from build123d import *

# Parameters (mm, degrees)
TUBE_SQUARE_40_X_40_X_3_2_1_DEPTH = 1920
CUT_EXTRUDE1_DEPTH                = 1921.52076271
SKETCH16_R                        = 2
CUT_EXTRUDE2_DEPTH                = 3
SKETCH17_R                        = 2
CUT_EXTRUDE3_DEPTH                = 3


with BuildPart() as part:
    # Sketch15 → Tube (square) 40 X 40 X 3.2(1) (new body)
    with BuildSketch(Plane(origin=(0, 0, 0), x_dir=(-1, 0, 0), z_dir=(0, 1, 0))):
        with BuildLine():
            Line((-13.6, -20), (13.6, -20))
            ThreePointArc((13.6, -20), (18.1254834, -18.1254834), (20, -13.6))
            Line((20, -13.6), (20, 13.6))
            ThreePointArc((20, 13.6), (18.1254834, 18.1254834), (13.6, 20))
            Line((13.6, 20), (-13.6, 20))
            ThreePointArc((-13.6, 20), (-18.1254834, 18.1254834), (-20, 13.6))
            Line((-20, 13.6), (-20, -13.6))
            ThreePointArc((-20, -13.6), (-18.1254834, -18.1254834), (-13.6, -20))
        make_face()
        with BuildLine():
            Line((-13.6, -16.8), (13.6, -16.8))
            ThreePointArc((13.6, -16.8), (15.8627417, -15.8627417), (16.8, -13.6))
            Line((16.8, -13.6), (16.8, 13.6))
            ThreePointArc((16.8, 13.6), (15.8627417, 15.8627417), (13.6, 16.8))
            Line((13.6, 16.8), (-13.6, 16.8))
            ThreePointArc((-13.6, 16.8), (-15.8627417, 15.8627417), (-16.8, 13.6))
            Line((-16.8, 13.6), (-16.8, -13.6))
            ThreePointArc((-16.8, -13.6), (-15.8627417, -15.8627417), (-13.6, -16.8))
        make_face(mode=Mode.SUBTRACT)
    extrude(amount=TUBE_SQUARE_40_X_40_X_3_2_1_DEPTH)

    # Sketch13 → Cut-Extrude1 (cut, through all)
    with BuildSketch(Plane(origin=(0, 0, -20), x_dir=(-1, 0, 0), z_dir=(0, 0, -1))):
        Polygon((20, 1880), (-20, 1920), (20, 1920), align=None)
    extrude(amount=-CUT_EXTRUDE1_DEPTH, mode=Mode.SUBTRACT)

    # Sketch16 → Cut-Extrude2 (cut)
    with BuildSketch(Plane(origin=(20, 0, 0), x_dir=(0, 0, -1), z_dir=(1, 0, 0))):
        with Locations((0, 1900)):
            Circle(SKETCH16_R)
        with Locations((0, 1447)):
            Circle(SKETCH16_R)
        with Locations((0, 1067)):
            Circle(SKETCH16_R)
        with Locations((0, 687)):
            Circle(SKETCH16_R)
    extrude(amount=-CUT_EXTRUDE2_DEPTH, mode=Mode.SUBTRACT)

    # Sketch17 → Cut-Extrude3 (cut)
    with BuildSketch(Plane(origin=(0, 0, -20), x_dir=(-1, 0, 0), z_dir=(0, 0, -1))):
        with Locations((0, 687)):
            Circle(SKETCH17_R)
        with Locations((0, 937)):
            Circle(SKETCH17_R)
    extrude(amount=-CUT_EXTRUDE3_DEPTH, mode=Mode.SUBTRACT)


solid = part.part
For this review, take the finished solid that the model builds, in its own axes (mm). Round coordinates to 2 decimals unless told otherwise and drop trailing zeros. Loops run counter-clockwise (first coordinate to the right, second up) from the corner with the lowest first, then second, coordinate; pieces in that order, holes last. Notation, with made-up numbers: (70, 35) - (129, 35) arc R13 ccw to (129, 54) - close; hole circle Ø10 at (47, 67). An arc over 180 degrees is marked (long way). Answer as CSV lines item,"result".
(1) Insertion check: P1, Ø2, axis at x = 1, y = 937.5, coming from the -Z side; P2, Ø6, axis at x = -1, z = -15.5, coming from the +Y side; P3, Ø3, axis at y = 1900, z = 0, coming from the -X side; P4, Ø2, axis at y = 1899.5, z = 0, coming from the +X side. Each pin has a flat end and moves straight along its axis. Give the tip position at first contact, or say it passes through.
Checked values:
P1,"stops at z = -20"
P2,"stops at y = 1901.7"
P3,"stops at x = 16.8"
P4,"stops at x = 17"
(2) Wall thickness on line 1 (Z direction, x = -6.5, y = 1326); line 2 (Y direction, x = 18, z = 0): over which ranges is each line inside the solid? List them lowest first.
Checked values:
line 1,"z = -20 to -16.8, 16.8 to 20"
line 2,"y = 0 to 685, 689 to 1065, 1069 to 1445, 1449 to 1898, 1902 to 1918"
(3) Consider section A-A on y = 613. Give the boundary of the cut face in (x, z).
Checked values:
outline,"(-20, -13.6) arc R6.4 ccw to (-13.6, -20) - (13.6, -20) arc R6.4 ccw to (20, -13.6) - (20, 13.6) arc R6.4 ccw to (13.6, 20) - (-13.6, 20) arc R6.4 ccw to (-20, 13.6) - close; hole (-16.8, -13.6) arc R3.2 ccw to (-13.6, -16.8) - (13.6, -16.8) arc R3.2 ccw to (16.8, -13.6) - (16.8, 13.6) arc R3.2 ccw to (13.6, 16.8) - (-13.6, 16.8) arc R3.2 ccw to (-16.8, 13.6) - close"
